Geometry check sheet. Reference: drawing and pictorial views, mm from the part's lowest x, y, z. A direction names the side the tool comes from. Coordinates: 2 decimals unless noted, no trailing zeros. Write each loop counter-clockwise with the first axis right and the second up, starting at its lowest first coordinate (ties: lowest second). Pieces come first, ordered by that corner, then holes. Notation, with made-up numbers: (52, 32.5) -> (82, 32.5) arc R9 cw to (82, 37.5) -> close; hole circle Ø5 at (16, 19.25). An arc over 180 degrees is marked (long way). Use a Markdown table: item, result.
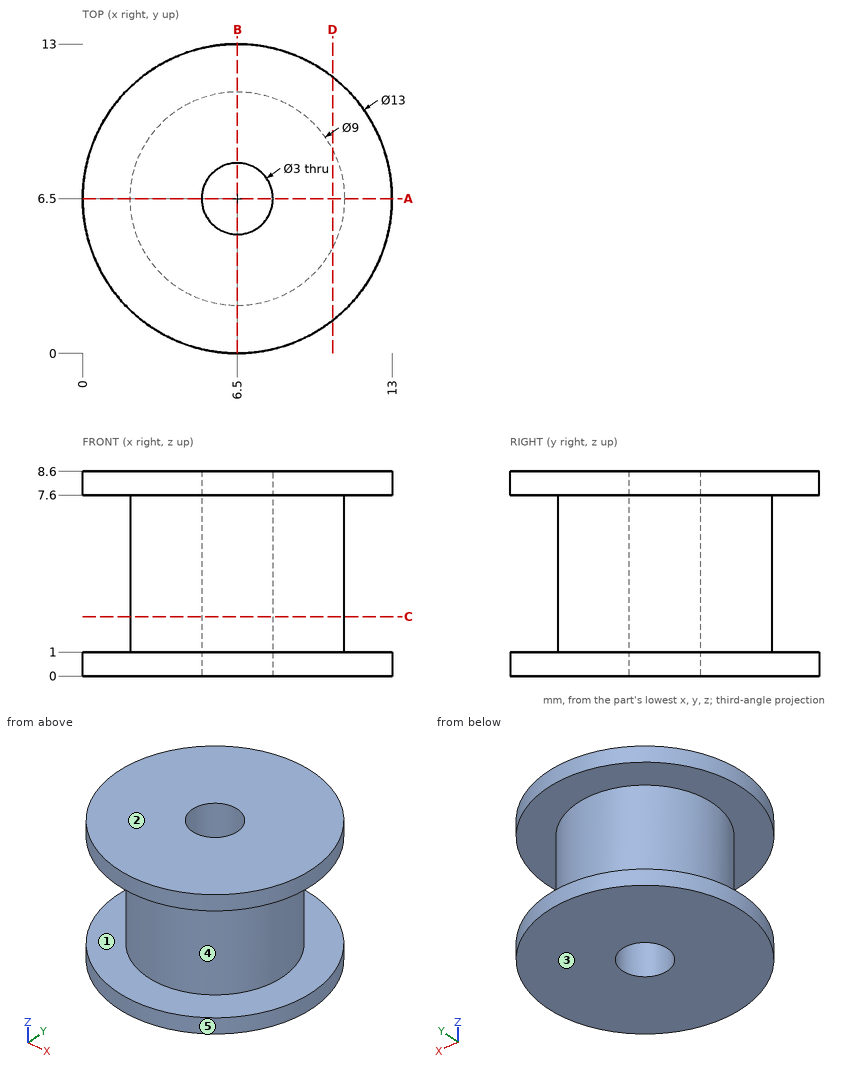
Item 1: Section check D-D on x = 10.5. Record the boundary of the cut face in (y, z).
Answer block:
| item | result |
|---|---|
| outline | (1.38, 0) -> (11.62, 0) -> (11.62, 1) -> (8.56, 1) -> (8.56, 7.6) -> (11.62, 7.6) -> (11.62, 8.6) -> (1.38, 8.6) -> (1.38, 7.6) -> (4.44, 7.6) -> (4.44, 1) -> (1.38, 1) -> close |
Item 2: Depth check by flat-ended pin: P1, Ø3.5, axis at x = 6.5, y = 6.5, coming from the +Z side; P2, Ø2, axis at y = 9.5, z = 3, coming from the +X side; P3, Ø3, axis at y = 3.5, z = 7, coming from the -X side. Enter the tip coordinate at first touch or a pass-through.
Answer block:
| item | result |
|---|---|
| P1 | stops at z = 8.6 |
| P2 | stops at x = 10.53 |
| P3 | stops at x = 0.21 |
Item 3: Mould release check, pull along Z, two halves, no side actions. Record for the marked faces 3, 4 and 5: +Z half, -Z half, draft (parallel to the pull), parting line (faces both ways), or undercut.
Answer block:
| item | result |
|---|---|
| face 3 | -Z half |
| face 4 | undercut |
| face 5 | draft |
Item 4: Tool access check on the marked faces 1 and 2. Record the directions out of +Z, -Z, +X, -X, +Y, -Y that give a thin tool (end or side, any length) a straight path to the whole face; none if there is none.
Answer block:
| item | result |
|---|---|
| face 1 | none |
| face 2 | +Z, +X, -X, +Y, -Y |
Item 5: Section check A-A on y = 6.5. Record the boundary of the cut face in (x, z).
Answer block:
| item | result |
|---|---|
| outline | (0, 0) -> (5, 0) -> (5, 8.6) -> (0, 8.6) -> (0, 7.6) -> (2, 7.6) -> (2, 1) -> (0, 1) -> close; (8, 0) -> (13, 0) -> (13, 1) -> (11, 1) -> (11, 7.6) -> (13, 7.6) -> (13, 8.6) -> (8, 8.6) -> close |
Item 6: Thickness scan on L1, parallel to Z at x = 7.75, y = 11.25; L2, parallel to Y at x = 6.5, z = 2.25; L3, parallel to Y at x = 7, z = 6.75. Record the ranges inside material, lowest first. Write a range as [from, to].
Answer block:
| item | result |
|---|---|
| L1 | z = [0, 1], [7.6, 8.6] |
| L2 | y = [2, 5], [8, 11] |
| L3 | y = [2.03, 5.09], [7.91, 10.97] |
Item 7: Section check C-C on z = 2.5. Record the boundary of the cut face in (x, y).
Answer block:
| item | result |
|---|---|
| outline | circle Ø9 at (6.5, 6.5); hole circle Ø3 at (6.5, 6.5) |
